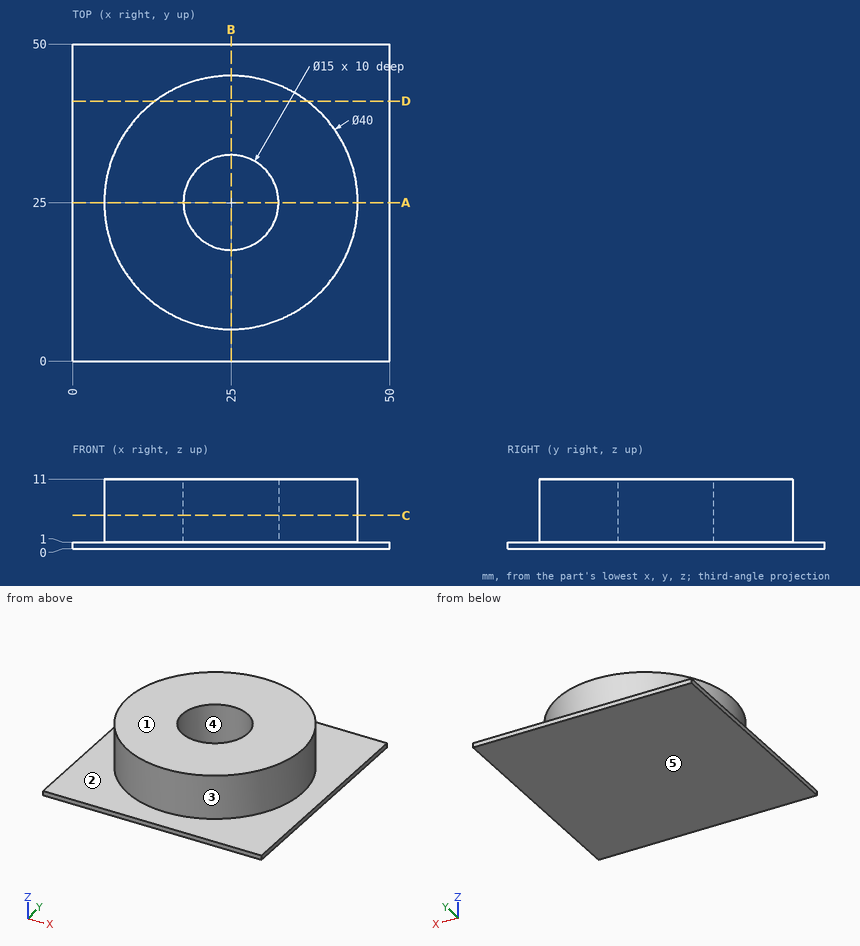
The figure shows three views and two pictorial views of one solid part (mm, origin at its lowest corner). Answer the questions. A direction names the side the tool comes from. Round coordinates to 2 decimals unless told otherwise and drop trailing zeros. Write each loop counter-clockwise with the first axis right and the second up, starting at its lowest first coordinate (ties: lowest second). Pieces come first, ordered by that corner, then holes. Notation, with made-up numbers: M 78.5,1 L 85.5,1 A12 cw 85.5,23 Z; hole C 39,-38.75 d11. An arc over 180 degrees is marked long. Use a Markdown table: item, result.
1) Consider line 1 (Y direction, x = 25, z = 4); line 2 (Z direction, x = 43.5, y = 12); line 3 (X direction, y = 22.5, z = 4.25). Determine where each line is inside the solid, lowest interval first. Write a range as [from, to].
Taken from the geometry:
| item | result |
|---|---|
| line 1 | y = [5, 17.5], [32.5, 45] |
| line 2 | z = [0, 1] |
| line 3 | x = [5.16, 17.93], [32.07, 44.84] |
2) Flat-ended cylindrical pins translate along their axes: pin 1 (2 mm diameter, centred on x = 5.5, z = 8.5, fed in from -Y); pin 2 (1.5 mm diameter, centred on x = 10, z = 5, fed in from -Y); pin 3 (12 mm diameter, centred on x = 25, y = 25, fed in from +Z). Find the tip coordinate at first contact, or state that the pin passes through.
Taken from the geometry:
| item | result |
|---|---|
| pin 1 | stops at y = 17.4 |
| pin 2 | stops at y = 10.97 |
| pin 3 | stops at z = 1 |
3) Determine the mould class of the marked faces 3, 4 and 5 for opening direction Y: pulls with the +Y half, pulls with the -Y half, needs draft (parallel to the pull), parting line crosses it, or undercut.
Taken from the geometry:
| item | result |
|---|---|
| face 3 | parting line crosses it |
| face 4 | undercut |
| face 5 | needs draft |
4) The part is cut by section D-D on y = 41. Give the vertices of the cut face in (x, z).
Taken from the geometry:
| item | result |
|---|---|
| outline | M 0,0 L 50,0 L 50,1 L 37,1 L 37,11 L 13,11 L 13,1 L 0,1 Z |
5) The part is cut by section C-C on z = 5.25. Give the vertices of the cut face in (x, y), plus the area to 3 significant figures.
Taken from the geometry:
| item | result |
|---|---|
| outline | C 25,25 d40; hole C 25,25 d15 |
| area | 1,080 mm2 |
6) The part is cut by section A-A on y = 25. Give the vertices of the cut face in (x, z).
Taken from the geometry:
| item | result |
|---|---|
| outline | M 0,0 L 50,0 L 50,1 L 45,1 L 45,11 L 32.5,11 L 32.5,1 L 17.5,1 L 17.5,11 L 5,11 L 5,1 L 0,1 Z |
7) Which of the six approach directions +Z, -Z, +X, -X, +Y, -Y give full straight-line access (tool end or side, diameter ignored) to the marked faces 1 and 2?
Taken from the geometry:
| item | result |
|---|---|
| face 1 | +Z, +X, -X, +Y, -Y |
| face 2 | +Z |
